Work out the finished part from the listing and answer in its coordinate system (mm). A direction names the side the tool comes from. Round coordinates to 2 decimals unless told otherwise and drop trailing zeros. Order: outer loops, then holes, each group sorted by start corner. A loop starts at its lowest first (then second) coordinate and runs counter-clockwise, first axis right, second up. Notation, with made-up numbers: (15, 23) - (54, 23) arc R37 ccw to (54, 61) - close; hole circle Ø11 at (-32, 88.25). An arc over 180 degrees is marked (long way). Answer in a Markdown table with one row per item.
from build123d import *

# Parameters (mm, degrees)
SKETCH_W        = 60
SKETCH_H        = 88
PAD_DEPTH       = 36
SKETCH001_W     = 48
SKETCH001_H     = 47.080017
POCKET_DEPTH    = 24
SKETCH002_W     = 24
SKETCH002_H     = 11.400024
POCKET001_DEPTH = 42.001
SKETCH003_W     = 18
SKETCH003_H     = 12
POCKET002_DEPTH = 10
POCKET003_DEPTH = 60.001
POCKET004_DEPTH = 7
POCKET005_DEPTH = 8
SKETCH007_W     = 24
SKETCH007_H     = 25.720013
POCKET006_DEPTH = 18


with BuildPart() as part:
    # Sketch → Pad (new body)
    with BuildSketch(Plane.XY):
        Rectangle(SKETCH_W, SKETCH_H)
    extrude(amount=PAD_DEPTH)

    # Sketch001 → Pocket (cut)
    with BuildSketch(Plane.XY.offset(36)):
        with Locations((0, -21.540008)):
            Rectangle(SKETCH001_W, SKETCH001_H)
    extrude(amount=-POCKET_DEPTH, mode=Mode.SUBTRACT)

    # Sketch002 → Pocket001 (cut, through all)
    with BuildSketch(Plane.XZ.offset(-2)):
        with Locations((0, 35.700012)):
            Rectangle(SKETCH002_W, SKETCH002_H)
    extrude(amount=-POCKET001_DEPTH, mode=Mode.SUBTRACT)

    # Sketch003 → Pocket002 (cut)
    with BuildSketch(Plane(origin=(-30, 0, 0), x_dir=(0, -1, 0), z_dir=(-1, 0, 0))):
        with Locations((25, 24)):
            Rectangle(SKETCH003_W, SKETCH003_H)
    extrude(amount=-POCKET002_DEPTH, mode=Mode.SUBTRACT)

    # Sketch004 → Pocket003 (cut, through all)
    with BuildSketch(Plane.YZ.offset(30)):
        Polygon((-50.809662, 9.705063), (-34, 0), (-50.809662, 0), align=None)
    extrude(amount=-POCKET003_DEPTH, mode=Mode.SUBTRACT)

    # Sketch005 → Pocket004 (cut)
    with BuildSketch(Plane.YZ.offset(30)):
        Polygon((-22, 12), (2, 30), (2, 12), align=None)
    extrude(amount=-POCKET004_DEPTH, mode=Mode.SUBTRACT)

    # Sketch006 → Pocket005 (cut)
    with BuildSketch(Plane.YZ.offset(30)):
        Polygon((-44, 36), (-44, 18), (-26, 36), align=None)
    extrude(amount=-POCKET005_DEPTH, mode=Mode.SUBTRACT)

    # Sketch007 → Pocket006 (cut)
    with BuildSketch(Plane.YZ.offset(30)):
        with Locations((20, 24.860007)):
            Rectangle(SKETCH007_W, SKETCH007_H)
    extrude(amount=-POCKET006_DEPTH, mode=Mode.SUBTRACT)


solid = part.part
1) Find section C-C, the plane y = -17.5. Give the vertices of the cut face in (x, z) (3 decimals), then the cut area to 3 significant figures.
Filled in:
| item | result |
|---|---|
| outline | (-30, 0) - (30, 0) - (30, 12) - (-24, 12) - (-24, 18) - (-30, 18) - close; (-30, 30) - (-24, 30) - (-24, 36) - (-30, 36) - close; (24, 15.375) - (30, 15.375) - (30, 36) - (24, 36) - close |
| area | 916 mm^2 |
2) Find section A-A, the plane z = 19.5. Give the vertices of the cut face in (x, y).
Filled in:
| item | result |
|---|---|
| outline | (-30, -44) - (-24, -44) - (-24, -34) - (-30, -34) - close; (-30, -16) - (-24, -16) - (-24, 2) - (30, 2) - (30, 8) - (12, 8) - (12, 32) - (30, 32) - (30, 44) - (-30, 44) - close; (24, -42.5) - (30, -42.5) - (30, -12) - (24, -12) - close |
3) The mould has two halves that part along X. Classify faces 5 (the face through (-12, 23, 33)), 6 (the face through (21, 38, 36)), 7 (the face through (-30, -1, 18)), 8 (the face through (30, -1, 10)): released by +X, released by -X, zero draft, split by the parting line, or undercut.
Filled in:
| item | result |
|---|---|
| face 5 | undercut |
| face 6 | zero draft |
| face 7 | released by -X |
| face 8 | released by +X |
4) Which of the six approach directions +Z, -Z, +X, -X, +Y, -Y give full straight-line access (tool end or side, diameter ignored) to faces 1 (the face through (0, 23, 30)), 2 (the face through (-27, -16, 24)), 3 (the face through (21, 32, 24)), 4 (the face through (24, -21, 24))?
Filled in:
| item | result |
|---|---|
| face 1 | +Z, +Y, -Y |
| face 2 | -X |
| face 3 | +Z, +X |
| face 4 | +Z, -Y |
5) Find the intervals of material crossed by probe 1 along Y at (x, z) = (19.5, 16.5); probe 2 along Y at (x, z) = (-26, 19); probe 3 along X at (y, z) = (-27.5, 17), in increasing order. Write a range as from..to.
Filled in:
| item | result |
|---|---|
| probe 1 | y = 2..8, 32..44 |
| probe 2 | y = -44..-34, -16..44 |
| probe 3 | x = -30..-24, 24..30 |
6) Find section B-B, the plane y = -30. Give the vertices of the cut face in (x, z).
Filled in:
| item | result |
|---|---|
| outline | (-30, 0) - (30, 0) - (30, 32) - (24, 32) - (24, 12) - (-24, 12) - (-24, 18) - (-30, 18) - close; (-30, 30) - (-24, 30) - (-24, 36) - (-30, 36) - close |
7) Find section D-D, the plane x = -4. Give the vertices of the cut face in (y, z).
Filled in:
| item | result |
|---|---|
| outline | (-44, 5.77) - (-34, 0) - (44, 0) - (44, 30) - (2, 30) - (2, 12) - (-44, 12) - close |
8) Each of these flat-tipped pins is pushed along its axis until it touches: pin 1 (12 mm diameter, centred on y = -24.5, z = 21.5, fed in from -X); pin 2 (20 mm diameter, centred on x = 23, z = 29.5, fed in from -Y); pin 3 (9 mm diameter, centred on x = 24, y = 25, fed in from +Z); pin 4 (9 mm diameter, centred on y = 16.5, z = 21, fed in from +X). Where does it stop, or does it pass through?
Filled in:
| item | result |
|---|---|
| pin 1 | stops at x = -30 |
| pin 2 | stops at y = -42.45 |
| pin 3 | stops at z = 12 |
| pin 4 | stops at x = 12 |
